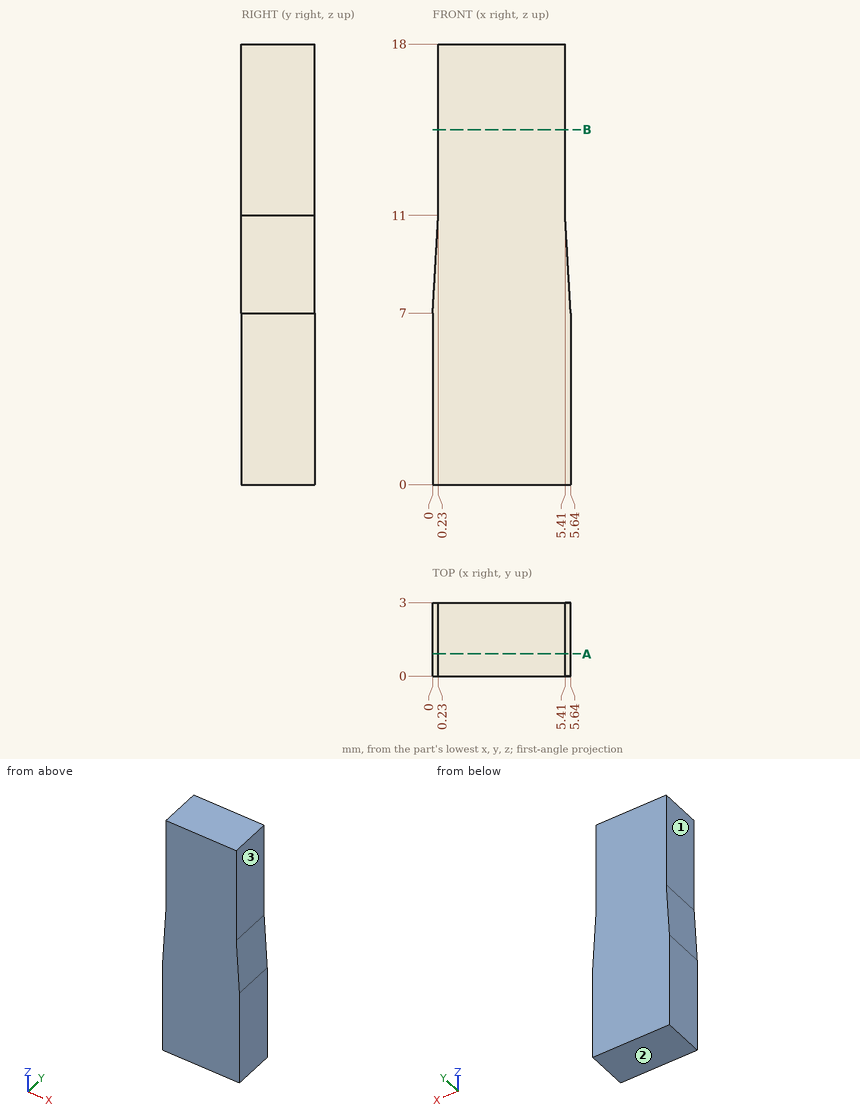
Verification items for this drawing (mm, ordinates from the low corner). A direction names the side the tool comes from. Give positions to 0.01 mm unless a question says otherwise; leave off trailing zeros. Write each loop counter-clockwise with the first axis right and the second up, starting at its lowest first coordinate (ties: lowest second). Pieces come first, ordered by that corner, then holes. Notation, with made-up numbers: (80.5, 7.25) - (86.5, 7.25) arc R22 cw to (86.5, 27.25) - close; hole circle Ø5 at (6.5, 77). An arc over 180 degrees is marked (long way). Answer as CSV lines item,"result". Start each with the question number.
1. Set-up check for the marked faces 1, 2 and 3: record each of +Z, -Z, +X, -X, +Y, -Y from which the full face is reachable in a straight line by a thin tool's end or side.
2. Sectioned sample at A-A (y = 0.9). Record the boundary of the cut face in (x, z).
3. Depth check by flat-ended pin: pin 1 (1.5 mm diameter, centred on y = 1.5, z = 13, fed in from -X). Enter the tip coordinate at first touch or a pass-through.
4. Thickness scan on line 1 (X direction, y = 1.8, z = 14.75); line 2 (X direction, y = 1.6, z = 8.75). Record the ranges inside material, lowest first.
5. Sectioned sample at B-B (z = 14.5). Record the boundary of the cut face in (x, y).
Derived:
1,face 1,"+Z, -X, +Y, -Y"
1,face 2,"-Z, +X, -X, +Y, -Y"
1,face 3,"+Z, +X, +Y, -Y"
2,outline,"(0, 0) - (5.64, 0) - (5.64, 7) - (5.41, 11) - (5.41, 18) - (0.23, 18) - (0.23, 11) - (0, 7) - close"
3,pin 1,"x = 0.23"
4,line 1,"0.23 to 5.41"
4,line 2,"0.1 to 5.54"
5,outline,"(0.23, 0) - (5.41, 0) - (5.41, 3) - (0.23, 3) - close"
